Read the model definition and answer for the solid it produces. Units are mm, in the model's axes. A direction names the side the tool comes from. Give positions to 0.01 mm unless a question says otherwise; leave off trailing zeros. Write each loop counter-clockwise with the first axis right and the second up, starting at its lowest first coordinate (ties: lowest second). Pieces come first, ordered by that corner, then holes.
```python
from build123d import *

# Parameters (mm, degrees)
SKETCH1_R           = 5
SKETCH1_R_2         = 1.65
BOSS_EXTRUDE1_DEPTH = 1
SKETCH1_3_R         = 3.9
SKETCH1_3_R_2       = 2.5
BOSS_EXTRUDE2_DEPTH = 10
SKETCH1_4_R         = 2.5
SKETCH1_4_R_2       = 1.65
BOSS_EXTRUDE3_DEPTH = 8


with BuildPart() as part:
    # Sketch1 → Boss-Extrude1 (new body)
    with BuildSketch(Plane.XY):
        Circle(SKETCH1_R)
        Circle(SKETCH1_R_2, mode=Mode.SUBTRACT)
    extrude(amount=-BOSS_EXTRUDE1_DEPTH)

    # Sketch1<3> → Boss-Extrude2 (add)
    with BuildSketch(Plane.XY):
        Circle(SKETCH1_3_R)
        Circle(SKETCH1_3_R_2, mode=Mode.SUBTRACT)
    extrude(amount=BOSS_EXTRUDE2_DEPTH)

    # Sketch1<4> → Boss-Extrude3 (add)
    with BuildSketch(Plane.XY):
        Circle(SKETCH1_4_R)
        Circle(SKETCH1_4_R_2, mode=Mode.SUBTRACT)
    extrude(amount=BOSS_EXTRUDE3_DEPTH)


solid = part.part
```
Item 1: Determine the mould class of faces 1 (the cylindrical face through (-1.216, 1.115, 3.437)), 2 (the cylindrical face through (-1.08, -4.88, -0.49)), 3 (the flat face through (3, -3, 0)) for opening direction Y: pulls with the +Y half, pulls with the -Y half, needs draft (parallel to the pull), parting line crosses it, or undercut.
Result set:
face 1: undercut
face 2: parting line crosses it
face 3: needs draft
Item 2: Section A-A (x = 0) is taken. Write down the section's boundary in (y, z), and give its area (3 significant figures).
Result set:
outline: (-5, -1) - (-1.65, -1) - (-1.65, 8) - (-2.5, 8) - (-2.5, 10) - (-3.9, 10) - (-3.9, 0) - (-5, 0) - close; (1.65, -1) - (5, -1) - (5, 0) - (3.9, 0) - (3.9, 10) - (2.5, 10) - (2.5, 8) - (1.65, 8) - close
area: 48.3 mm2
Item 3: Section C-C (z = 3.25) is taken. Write down the section's boundary in (x, y), and give its area (3 significant figures).
Result set:
outline: circle Ø7.8 at (0, 0); hole circle Ø3.3 at (0, 0)
area: 39.2 mm2
Item 4: Find the intervals of material crossed by line 1 along Y through (x, z) = (0, 9.35); line 2 along Y through (x, z) = (0, 3); line 3 along Z through (x, y) = (1, 4), in increasing order.
Result set:
line 1: y = -3.9 to -2.5, 2.5 to 3.9
line 2: y = -3.9 to -1.65, 1.65 to 3.9
line 3: z = -1 to 0
Item 5: Each of these flat-tipped pins is pushed along its axis until it touches: pin 1 Ø4.5 at (x, y) = (0, 0) entering from +Z; pin 2 Ø2 at (x, y) = (0, 0) entering from -Z; pin 3 Ø5 at (y, z) = (-1, 5.5) entering from -X; pin 4 Ø3 at (x, z) = (-3, 5) entering from -Y. Where does it stop, or does it pass through?
Result set:
pin 1: stops at z = 8
pin 2: passes through
pin 3: stops at x = -3.9
pin 4: stops at y = -3.6
Item 6: Section D-D (x = 4.25) is taken. Write down the section's boundary in (y, z), and give its area (3 significant figures).
Result set:
outline: (-2.63, -1) - (2.63, -1) - (2.63, 0) - (-2.63, 0) - close
area: 5.27 mm2
Item 7: Which of the six approach directions +Z, -Z, +X, -X, +Y, -Y give full straight-line access (tool end or side, diameter ignored) to faces 4 (the flat face through (0, -3, 10)), 5 (the flat face through (2, -1, 8))?
Result set:
face 4: +Z, +X, -X, +Y, -Y
face 5: +Z
